Autodesk Inventor part; units mm, degrees
ref_plane "YZ Plane" through (0, 0, 0) normal (1, 0, 0) x (0, 1, 0)
ref_plane "XZ Plane" through (0, 0, 0) normal (0, 1, 0) x (-1, 0, 0)
ref_plane "XY Plane" through (0, 0, 0) normal (0, 0, 1) x (1, 0, 0)
sketch "Szkic1" plane through (0, 0, 0) normal (0, 0, 1) x (1, 0, 0)
  line L0 (6, -2.25) -> (-6, -2.25)
  line L1 (-6, -2.25) -> (-6, 2.25)
  line L2 (-6, 2.25) -> (6, 2.25)
  line L3 (6, 2.25) -> (6, -2.25)
  line L4 (6, -2.25) -> (-6, 2.25) construction
  line L5 (-6, -2.25) -> (6, 2.25) construction
  line L6 (6, -2.25) -> (-6, -2.25)
  line L7 (-6, -2.25) -> (-6, 2.25)
  line L8 (-6, 2.25) -> (6, 2.25)
  line L9 (6, 2.25) -> (6, -2.25)
  line L10 (6, -2.25) -> (-6, 2.25) construction
  line L11 (-6, -2.25) -> (6, 2.25) construction
  point P0 (0, 0)
  dimension "d0" = 12
  dimension "d1" = 4.5
extrude "Wyciągnięcie proste1" add sketch "Szkic1" against normal blind 10
sketch "Szkic2" plane through (0, 0, -10) normal (0, 0, -1) x (-1, 0, 0)
  line L0 (6, 2.25) -> (-6, 2.25)
  line L1 (6, -2.25) -> (-6, -2.25)
  line L2 (-6, -2.25) -> (-6, 2.25)
  line L3 (-6, 2.25) -> (6, 2.25)
  line L4 (6, 2.25) -> (6, -2.25)
  line L5 (6, -2.25) -> (-6, 2.25) construction
  line L6 (-6, -2.25) -> (6, 2.25) construction
  point P0 (0, 0)
sketch "Szkic3" plane through (0, 0, 0) normal (0, 0, 1) x (1, 0, 0)
  line L0 (10, -6.25) -> (-10, -6.25)
  line L1 (-10, -6.25) -> (-10, 6.25)
  line L2 (-10, 6.25) -> (10, 6.25)
  line L3 (10, 6.25) -> (10, -6.25)
  line L4 (10, -6.25) -> (-10, 6.25) construction
  line L5 (-10, -6.25) -> (10, 6.25) construction
  point P0 (0, 0)
  dimension "d4" = 20
  dimension "d5" = 12.5
extrude "Wyciągnięcie proste2" add sketch "Szkic3" along normal blind 20
sketch "Szkic5" plane through (0, 0, 20) normal (0, 0, 1) x (1, 0, 0)
  line L0 (15, -7.75) -> (-15, -7.75)
  line L1 (-15, -7.75) -> (-15, 7.75)
  line L2 (-15, 7.75) -> (15, 7.75)
  line L3 (15, 7.75) -> (15, -7.75)
  line L4 (15, -7.75) -> (-15, 7.75) construction
  line L5 (-15, -7.75) -> (15, 7.75) construction
  point P0 (0, 0)
  dimension "d8" = 15.5
  dimension "d9" = 30
extrude "Wyciągnięcie proste3" add sketch "Szkic5" along normal blind 35
sketch "Szkic6" plane through (0, 0, 55) normal (0, 0, 1) x (1, 0, 0)
  line L0 (17.5, -10) -> (-17.5, -10)
  line L1 (-17.5, -10) -> (-17.5, 10)
  line L2 (-17.5, 10) -> (17.5, 10)
  line L3 (17.5, 10) -> (17.5, -10)
  line L4 (17.5, -10) -> (-17.5, 10) construction
  line L5 (-17.5, -10) -> (17.5, 10) construction
  point P0 (0, 0)
  dimension "d12" = 20
  dimension "d13" = 35
extrude "Wyciągnięcie proste4" add sketch "Szkic6" along normal blind 25
sketch "Szkic7" plane through (0, 0, 80) normal (0, 0, 1) x (1, 0, 0)
  line L0 (15, -5) -> (-15, -5)
  line L1 (-15, -5) -> (-15, 5)
  line L2 (-15, 5) -> (15, 5)
  line L3 (15, 5) -> (15, -5)
  line L4 (15, -5) -> (-15, 5) construction
  line L5 (-15, -5) -> (15, 5) construction
  point P0 (0, 0)
  dimension "d16" = 10
  dimension "d17" = 30
extrude "Wyciągnięcie proste5" add sketch "Szkic7" along normal blind 5
fillet "Zaokrąglenie1" radius 2 4 edges at (0, 10, 55) (-17.5, 0, 55) (17.5, 0, 55) (0, -10, 55)
fillet "Zaokrąglenie2" radius 2 8 edges at (16.9142, 9.4142, 55.5858) (17.5, 10, 68.5) (-16.9142, 9.4142, 55.5858) (-17.5, 10, 68.5) (16.9142, -9.4142, 55.5858) (17.5, -10, 68.5) (-16.9142, -9.4142, 55.5858) (-17.5, -10, 68.5)
properties part number "USB2Dynamixel-XD"
Input: part model. Units: mm. Frame: model coordinates. A direction names the side the tool comes from. Give positions to 0.01 mm unless a question says otherwise; leave off trailing zeros. Write each loop counter-clockwise with the first axis right and the second up, starting at its lowest first coordinate (ties: lowest second). Pieces come first, ordered by that corner, then holes.
Q1. Section B-B, the plane y = -0.5. Output: boundary loops of the cut face in (x, z).
Q2. Set-up query: faces 1 (the face through (0, -2.25, -5)), 2 (the face through (15, 0, 37)), 3 (the face through (0, -5, 82)), 4 (the face through (0, 6.25, 10)), 5 (the face through (0, 5, 82)). Return all of +Z, -Z, +X, -X, +Y, -Y with unobstructed straight access to the full face (end or side cutting, diameter ignored); none if empty.
Q3. Section A-A, the plane x = 3. Output: boundary loops of the cut face in (y, z), plus the area to 3 significant figures.
Q4. Material intervals for probe 1 along Z at (x, y) = (7.5, 1.5); probe 2 along Y at (x, z) = (10, 28); probe 3 along X at (y, z) = (1.75, -2), sorted ascending.
Q5. First-contact query: P1, Ø2, axis at x = 5, z = 27.5, coming from the +Y side; P2, Ø10, axis at y = -1.5, z = 6.5, coming from the -X side; P3, Ø4, axis at x = 2, y = -3, coming from the -Z side; P4, Ø1.5, axis at y = -1, z = 83.5, coming from the -X side. Flat tips, straight axial feed; report the tip coordinate or a pass-through.
Q6. Section D-D, the plane x = 8. Output: boundary loops of the cut face in (y, z), plus the area to 3 significant figures.
Q7. Section C-C, the plane z = 47. Output: boundary loops of the cut face in (x, y).
Filled in:
1. outline: (-17.5, 57) arc R2 ccw to (-15.5, 55) - (-15, 55) - (-15, 20) - (-10, 20) - (-10, 0) - (-6, 0) - (-6, -10) - (6, -10) - (6, 0) - (10, 0) - (10, 20) - (15, 20) - (15, 55) - (15.5, 55) arc R2 ccw to (17.5, 57) - (17.5, 80) - (15, 80) - (15, 85) - (-15, 85) - (-15, 80) - (-17.5, 80) - close
2. face 1: -Z, +X, -X, -Y
2. face 2: -Z, +X, +Y, -Y
2. face 3: +Z, +X, -X, -Y
2. face 4: -Z, +X, -X, +Y
2. face 5: +Z, +X, -X, +Y
3. outline: (-10, 57) arc R2 ccw to (-8, 55) - (-7.75, 55) - (-7.75, 20) - (-6.25, 20) - (-6.25, 0) - (-2.25, 0) - (-2.25, -10) - (2.25, -10) - (2.25, 0) - (6.25, 0) - (6.25, 20) - (7.75, 20) - (7.75, 55) - (8, 55) arc R2 ccw to (10, 57) - (10, 80) - (5, 80) - (5, 85) - (-5, 85) - (-5, 80) - (-10, 80) - close
3. area: 1,390 mm2
4. probe 1: z = 0 to 85
4. probe 2: y = -7.75 to 7.75
4. probe 3: x = -6 to 6
5. P1: stops at y = 7.75
5. P2: stops at x = -10
5. P3: stops at z = -10
5. P4: stops at x = -15
6. outline: (-10, 57) arc R2 ccw to (-8, 55) - (-7.75, 55) - (-7.75, 20) - (-6.25, 20) - (-6.25, 0) - (6.25, 0) - (6.25, 20) - (7.75, 20) - (7.75, 55) - (8, 55) arc R2 ccw to (10, 57) - (10, 80) - (5, 80) - (5, 85) - (-5, 85) - (-5, 80) - (-10, 80) - close
6. area: 1,340 mm2
7. outline: (-15, -7.75) - (15, -7.75) - (15, 7.75) - (-15, 7.75) - close
